from build123d import *

# Parameters (mm, degrees)
F0_W        = 66.1063343287
F0_H        = 38.1483472884
F1_DEPTH    = 1.27
F3_DEPTH    = 25.4
F4_T        = 1.27
F4_T3_DEPTH = 43.2463343287
F4_T5_DEPTH = 43.2463343287
F4_T7_DEPTH = 43.2463343287
F5_W        = 17.286144197
F5_H        = 6.7250733264
F6_DEPTH    = 1.27


# Not quite as in the source:
# - a shell that OpenCascade refuses in one call is made with other operations: the cavity is built on its own and cut out


with BuildPart() as f1:
    # F0 (on Top) → F1 (new body)
    with BuildSketch(Plane.XY):
        Rectangle(F0_W, F0_H)
    extrude(amount=F1_DEPTH)

    # F2 (on face) → F3 (join)
    with BuildSketch(Plane.XY.offset(1.27)):
        Polygon((20.3531671643, 16.5341736442), (-20.3531671643, 16.5341736442), (0, -18.7185459794), align=None)
    extrude(amount=F3_DEPTH)

    # F4: shell of thickness 1.27, made by hand


with BuildPart() as f4_core1:
    # F4_t2: copy of F1
    add(f1.part)

    # the walls: a layer under each face that stays
    f4_faces = [f4_core1.faces().sort_by_distance(p)[0] for p in [
        (33.0531671643, 0, 0.635),
        (0, -19.0741736442, 0.635),
        (0, 19.0741736442, 0.635),
        (0, 0, 0),
        (-22.0354447762, -12.7161157628, 1.27),
        (-33.0531671643, 0, 0.635),
        (0, 16.5341736442, 13.97),
        (-10.1765835822, -1.0921861676, 13.97),
        (10.1765835822, -1.0921861676, 13.97),
    ]]
    thicken(f4_faces, amount=-F4_T, mode=Mode.SUBTRACT)

    # F4_s4 → F4_t3 (cut)
    with BuildSketch(Plane.YZ.offset(-21.6231671643)):
        Polygon((16.5468736442, 1.2827), (16.5341736442, 0), (15.2641736442, 0), (15.2641736442, 1.27), align=None)
    extrude(amount=F4_T3_DEPTH, mode=Mode.SUBTRACT)

    # F4_s6 → F4_t5 (cut)
    with BuildSketch(Plane(origin=(-12.8827989943, 22.3136624018, 0), x_dir=(0, 0, 1), z_dir=(0.5, -0.8660254038, 0))):
        Polygon((1.2827, 9.3719729897), (0, 9.3592729897), (0, 8.0892729897), (1.27, 8.0892729897), align=None)
    extrude(amount=F4_T5_DEPTH, mode=Mode.SUBTRACT)

    # F4_s8 → F4_t7 (cut)
    with BuildSketch(Plane(origin=(-8.74036817, -15.1387617473, 0), x_dir=(0, 0, 1), z_dir=(0.5, 0.8660254038, 0))):
        Polygon((1.2827, 9.3719729897), (0, 9.3592729897), (0, 8.0892729897), (1.27, 8.0892729897), align=None)
    extrude(amount=F4_T7_DEPTH, mode=Mode.SUBTRACT)


with BuildPart() as f1_1:
    add(f1.part)

    # what is left inside the walls is the cavity
    f4_cavity = [f4_core1.part.solids().sort_by_distance(p)[0] for p in [
        (-9.065733, -0.450836, 18.203333),
    ]]
    add(f4_cavity, mode=Mode.SUBTRACT)

    # F5 (on face) → F6 (join)
    with BuildSketch(Plane.XY.offset(1.27)):
        with Locations((-19.0954133868, -9.2882269528)):
            Rectangle(F5_W, F5_H)
    extrude(amount=F6_DEPTH)


solid = f1_1.part
For this review, take the finished solid that the model builds, in its own axes (mm). A direction names the side the tool comes from. Coordinates: 2 decimals unless noted, no trailing zeros. Write each loop counter-clockwise with the first axis right and the second up, starting at its lowest first coordinate (ties: lowest second). Pieces come first, ordered by that corner, then holes. Notation, with made-up numbers: (48.5, 76) -> (98.5, 76) arc R16 ccw to (98.5, 87) -> close; hole circle Ø3 at (49.5, 42.25). An arc over 180 degrees is marked (long way). Write each question's results on one line, items separated by ' | '. Start each with the question number.
1) Wall thickness on L1, parallel to Y at x = -12.5, z = 2; L2, parallel to Z at x = 0.5, y = -4.5; L3, parallel to Z at x = -13, y = -9.5: over which ranges is each line inside the solid? List them lowest first. Write a range as [from, to].
2) Consider section A-A (x = -21). Write out the cut boundary in (y, z), plus the area to 3 significant figures.
3) For faces 5 (the face through (8.95, -0.68, 13.79)), 6 (the face through (-10.452, -9, 2)), 7 (the face through (-27.738, -9, 2)), 8 (the face through (-19, -12.651, 2)), list the 3-axis set-ups (+Z, -Z, +X, -X, +Y, -Y) from which the entire face can be reached by the end or side of a thin tool; tool diameter is ignored.
4) Insertion check: pin 1 (7.5 mm diameter, centred on x = -19, y = -10, fed in from +Z); pin 2 (8 mm diameter, centred on x = -11, z = 20, fed in from +Y); pin 3 (6 mm diameter, centred on x = 25, y = 13, fed in from +Z). Each pin has a flat end and moves straight along its axis. Give the tip position at first contact, or say it passes through.
5) Consider section C-C (y = -1.5). Write out the cut boundary in (x, z), plus the area to 3 significant figures.
6) Consider section B-B (z = 8.75). Write out the cut boundary in (x, y), plus the area to 3 significant figures.
7) The part is to be moulded in two halves that separate along Y. For faces 1 (the face through (0, 15.264, 14)), 2 (the face through (10.034, -1.339, 13.792)), 3 (the face through (0, 16.534, 14)), 4 (the face through (-19, -5.926, 2)), say which applies: +Y half, -Y half, draft (parallel to the pull), parting line (faces both ways), or undercut.
8) Consider section D-D (x = 23.5). Write out the cut boundary in (y, z), plus the area to 3 significant figures.
Geometry says:
1) L1: [-12.65, -5.93], [2.93, 5.47], [15.26, 16.53] | L2: [0, 1.27] | L3: [0, 2.54]
2) outline: (-19.07, 0) -> (19.07, 0) -> (19.07, 1.27) -> (-5.93, 1.27) -> (-5.93, 2.54) -> (-12.65, 2.54) -> (-12.65, 1.27) -> (-19.07, 1.27) -> close | area: 57.0 mm^2
3) face 5: +Z | face 6: +Z, -Y | face 7: +Z, -X, +Y, -Y | face 8: +Z, -X, -Y
4) pin 1: z = 2.54 | pin 2: y = 16.53 | pin 3: z = 1.27
5) outline: (-33.05, 0) -> (33.05, 0) -> (33.05, 1.27) -> (9.94, 1.27) -> (9.94, 26.67) -> (8.47, 26.67) -> (8.47, 1.27) -> (-8.47, 1.27) -> (-8.47, 26.67) -> (-9.94, 26.67) -> (-9.94, 1.27) -> (-33.05, 1.27) -> close | area: 158 mm^2
6) outline: (-20.35, 16.53) -> (0, -18.72) -> (20.35, 16.53) -> close; hole (-18.15, 15.26) -> (0, -16.18) -> (18.15, 15.26) -> close | area: 147 mm^2
7) face 1: undercut | face 2: -Y half | face 3: +Y half | face 4: undercut
8) outline: (-19.07, 0) -> (19.07, 0) -> (19.07, 1.27) -> (-19.07, 1.27) -> close | area: 48.4 mm^2
